Input: part model. Units: mm. Frame: model coordinates. A direction names the side the tool comes from. Coordinates: 2 decimals unless noted, no trailing zeros. Order: outer loops, then holes, each group sorted by start corner. A loop starts at its lowest first (then second) coordinate and runs counter-clockwise, first axis right, second up. Notation, with made-up numbers: (14.25, 85.25) -> (64.25, 85.25) arc R9 cw to (64.25, 95.25) -> close; hole circle Ø2 at (48.5, 76.5). An arc over 180 degrees is marked (long way). One line per item, written item: value. Start each with the question number.
from build123d import *

# Parameters (mm, degrees)
SKETCH1_W           = 25
SKETCH1_H           = 50
SKETCH1_R           = 3.4
BOSS_EXTRUDE1_DEPTH = 3
SKETCH2_W           = 50
SKETCH2_H           = 3
BOSS_EXTRUDE2_DEPTH = 8
SKETCH3_W           = 8
SKETCH3_H           = 50
BOSS_EXTRUDE3_DEPTH = 42
SKETCH4_R           = 2.65
CUT_EXTRUDE1_DEPTH  = 6.6
SKETCH5_R           = 5.802370205
CUT_EXTRUDE2_DEPTH  = 9
FILLET2_R           = 1
SKETCH6_R           = 12.6
BOSS_EXTRUDE4_DEPTH = 2
FILLET4_R           = 1
SKETCH8_R           = 1.589780168
SKETCH8_R_2         = 1.777428262
CUT_EXTRUDE3_DEPTH  = 10
SKETCH9_W           = 49.021678163
SKETCH9_H           = 20.976854622
CUT_EXTRUDE4_DEPTH  = 68.79439129


with BuildPart() as part:
    # Sketch1 → Boss-Extrude1 (new body)
    with BuildSketch(Plane(origin=(0, 0, 0), x_dir=(1, 0, 0), z_dir=(0, 1, 0))):
        with Locations((2.276951673, 11.384758364)):
            Rectangle(SKETCH1_W, SKETCH1_H)
        with Locations(Location((1.276951673, 11.384758364, 0), (0, 0, 270))):
            Circle(SKETCH1_R, mode=Mode.SUBTRACT)
    extrude(amount=BOSS_EXTRUDE1_DEPTH)

    # Sketch2 → Boss-Extrude2 (add)
    with BuildSketch(Plane.ZY.offset(10.223048327)):
        with Locations((-11.384758364, 1.5)):
            Rectangle(SKETCH2_W, SKETCH2_H)
    extrude(amount=BOSS_EXTRUDE2_DEPTH)

    # Sketch3 → Boss-Extrude3 (add)
    with BuildSketch(Plane.XZ):
        with Locations((-14.223048327, -11.384758364)):
            Rectangle(SKETCH3_W, SKETCH3_H)
    extrude(amount=BOSS_EXTRUDE3_DEPTH)

    # Sketch4 → Cut-Extrude1 (cut)
    with BuildSketch(Plane(origin=(0, 3, 0), x_dir=(1, 0, 0), z_dir=(0, 1, 0))):
        with Locations(Location((-14.223048327, 32.384758364, 0), (0, 0, 270))):
            Circle(SKETCH4_R)
        with Locations(Location((-14.223048327, -9.615241636, 0), (0, 0, 270))):
            Circle(SKETCH4_R)
    cut_extrude1 = extrude(amount=-CUT_EXTRUDE1_DEPTH, mode=Mode.SUBTRACT)

    # Mirror1: Cut-Extrude1 across plane
    add(cut_extrude1.mirror(Plane.ZX.offset(-19.5)), mode=Mode.SUBTRACT)

    # Sketch5 → Cut-Extrude2 (cut)
    with BuildSketch(Plane.ZY.offset(18.223048327)):
        with Locations((-11.836279124, -21)):
            Circle(SKETCH5_R)
    extrude(amount=-CUT_EXTRUDE2_DEPTH, mode=Mode.SUBTRACT)

    # Fillet2
    fillet2_edges = [part.edges().sort_by_distance(p)[0] for p in [
        (-10.223048327, -21, -17.638649329),
    ]]
    fillet(fillet2_edges, radius=FILLET2_R)

    # Mirror2: Cut-Extrude1 across plane
    add(cut_extrude1.mirror(Plane.ZY.offset(1.723048327)), mode=Mode.SUBTRACT)

    # Sketch6 → Boss-Extrude4 (add)
    with BuildSketch(Plane(origin=(0, 3, 0), x_dir=(1, 0, 0), z_dir=(0, 1, 0))):
        with BuildLine():
            Line((14.776951673, 5.825082115), (14.776951673, 16.944434614))
            ThreePointArc((14.776951673, 16.944434614), (-13.323048327, 11.384758364), (14.776951673, 5.825082115))
        make_face()
        with Locations(Location((1.276951673, 11.384758364, 0), (0, 0, 270))):
            Circle(SKETCH6_R, mode=Mode.SUBTRACT)
    extrude(amount=BOSS_EXTRUDE4_DEPTH)

    # Fillet4
    # the kernel refuses this fillet: 1 mm, written as the material it takes off along each edge
    with BuildSketch(Plane(origin=(14.776951673, 5, -3.325082115), x_dir=(0, -1, 0), z_dir=(0, 0, -1))) as fillet4_piece_1:
        with BuildLine():
            CenterArc((FILLET4_R, FILLET4_R), FILLET4_R, 180, 90)
            Line((0, FILLET4_R), (0, 0))
            Line((0, 0), (FILLET4_R, 0))
        make_face()
    extrude(amount=16.119352499, mode=Mode.SUBTRACT)

    # Sketch8 → Cut-Extrude3 (cut)
    with BuildSketch(Plane(origin=(0, 3, 0), x_dir=(1, 0, 0), z_dir=(0, 1, 0))):
        with Locations(Location((1.276951673, 19.884758364, 0), (0, 0, 270))):
            Circle(SKETCH8_R)
        with Locations(Location((1.276951673, 2.884758364, 0), (0, 0, 270))):
            Circle(SKETCH8_R_2)
    extrude(amount=-CUT_EXTRUDE3_DEPTH, mode=Mode.SUBTRACT)

    # Sketch9 → Cut-Extrude4 (cut, through all)
    with BuildSketch(Plane.XY.offset(13.615241636)):
        with Locations((-9.733887409, 10.488427311)):
            Rectangle(SKETCH9_W, SKETCH9_H)
    extrude(amount=-CUT_EXTRUDE4_DEPTH, mode=Mode.SUBTRACT)


solid = part.part
1) Section query A-A, the plane y = -21. Return the cut outline in (x, z), plus the area to 3 significant figures.
2) Section query C-C, the plane z = 7.5. Return the cut outline in (x, y), plus the area to 3 significant figures.
3) Pin query (flat end, axial travel): pin 1 Ø2.5 at (x, z) = (-14.5, 9) entering from -Y; pin 2 Ø2.5 at (x, z) = (-14.5, 8.5) entering from +Y. Return the tip coordinate at first contact, or that it passes through.
4) Section query D-D, the plane y = -38. Return the cut outline in (x, z).
5) Ray query, line 1 along Z through (x, y) = (-12.5, -3); line 2 along Y through (x, z) = (-15.75, -15); line 3 along Z through (x, y) = (-10.5, -19). Return the intervals inside material, ascending. Write a range as from..to.
6) Section query B-B, the plane x = -15.5. Return the cut outline in (y, z), plus the area to 3 significant figures.
7) Access query for faces 5 (the cylindrical face through (-11.99, -38.75, -30.96)), 6 (the cylindrical face through (-11.99, -1.77, -30.96)), 7 (the flat face through (-14, -21, 13.615)). Directions: +Z, -Z, +X, -X, +Y, -Y. A direction counts if a zero-diameter tool reaches every point of the face in a straight line with its end or side. Return the directions, or none.
8) Mould query, pull axis X, two halves, no side actions, for faces 1 (the cylindrical face through (-11.596, -38.746, 9.27)), 2 (the flat face through (-10.223, -16, -17)), 3 (the flat face through (-18.223, -16, -17)), 4 (the cylindrical face through (-14.772, -17.078, -16.113)). Classes: +X half, -X half, draft (parallel to the pull), parting line (faces both ways), or undercut.
Entries:
1. outline: (-18.22, -36.38) -> (-10.22, -36.38) -> (-10.22, -18.64) arc R1 ccw to (-11.22, -17.64) -> (-18.22, -17.64) -> close; (-18.22, -6.03) -> (-11.22, -6.03) arc R1 ccw to (-10.22, -5.03) -> (-10.22, 13.62) -> (-18.22, 13.62) -> close
1. area: 307 mm2
2. outline: (-18.22, -42) -> (-15.82, -42) -> (-15.82, -35.4) -> (-12.63, -35.4) -> (-12.63, -42) -> (-10.22, -42) -> (-10.22, 0) -> (-12.63, 0) -> (-12.63, -3.6) -> (-15.82, -3.6) -> (-15.82, 0) -> (-18.22, 0) -> close
2. area: 303 mm2
3. pin 1: stops at y = -35.4
3. pin 2: stops at y = -3.6
4. outline: (-18.22, -36.38) -> (-10.22, -36.38) -> (-10.22, 13.62) -> (-18.22, 13.62) -> close; hole circle Ø5.3 at (-14.22, -32.38); hole circle Ø5.3 at (-14.22, 9.62)
5. line 1: z = -36.38..-34.4, -30.37..7.6, 11.63..13.62
5. line 2: y = -42..-25.86, -16.14..0
5. line 3: z = -36.38..-17.61, -6.06..13.62
6. outline: (-42, -36.38) -> (0, -36.38) -> (0, -34.71) -> (-3.6, -34.71) -> (-3.6, -30.06) -> (0, -30.06) -> (0, 7.29) -> (-3.6, 7.29) -> (-3.6, 11.94) -> (0, 11.94) -> (0, 13.62) -> (-42, 13.62) -> (-42, 11.94) -> (-35.4, 11.94) -> (-35.4, 7.29) -> (-42, 7.29) -> (-42, -30.06) -> (-35.4, -30.06) -> (-35.4, -34.71) -> (-42, -34.71) -> close; hole circle Ø11.6 at (-21, -11.84)
6. area: 1,900 mm2
7. face 5: -Y
7. face 6: +Y
7. face 7: +Z, +X, -X, +Y, -Y
8. face 1: undercut
8. face 2: +X half
8. face 3: -X half
8. face 4: draft
